```python
from build123d import *

# Parameters (mm, degrees)
SKETCH1_W                           = 3.81
SKETCH1_H                           = 63.5
CUT_EXTRUDE1_REACH                  = 281.224
CUT_EXTRUDE1_END_RADIUS             = 142.71625
SKETCH2_W                           = 1.524
SKETCH2_H                           = 38.1
CUT_EXTRUDE1_DIRECTION_2_REACH      = 281.224
CUT_EXTRUDE1_DIRECTION_2_END_RADIUS = 142.71625
CIRPATTERN1_COUNT                   = 4
CIRPATTERN1_ANGLE                   = 135


with BuildPart() as part:
    # Sketch1 → Revolve1 (revolve)
    with BuildSketch(Plane.XY, mode=Mode.PRIVATE) as revolve1_sk:
        with Locations((140.81125, 161.201652174)):
            Rectangle(SKETCH1_W, SKETCH1_H)
    revolve(revolve1_sk.sketch.rotate(Axis((0, 0, 0), (0, -1, 0)), 90), axis=Axis((0, 0, 0), (0, -1, 0)))

    # Cut-Extrude1: up to this cylinder (the profile starts inside it)
    cut_extrude1_end = Plane(origin=(0, 161.201652, 0), z_dir=(0, 1, 0)) * Cylinder(CUT_EXTRUDE1_END_RADIUS, 848.8805, mode=Mode.PRIVATE)
    # Sketch2 → Cut-Extrude1 (cut, up to the surface)
    with BuildSketch(Plane(origin=(0, 0, 0), x_dir=(0, 0, -1), z_dir=(1, 0, 0)), mode=Mode.PRIVATE) as cut_extrude1_sk1:
        with Locations((0, 161.201652174)):
            Rectangle(SKETCH2_W, SKETCH2_H)
    cut_extrude1_tool1 = extrude(cut_extrude1_sk1.sketch, amount=-CUT_EXTRUDE1_REACH, mode=Mode.PRIVATE) & cut_extrude1_end
    cut_extrude1 = cut_extrude1_tool1.solids().sort_by_distance((0, 161.201652, 0))[0]
    add(cut_extrude1, mode=Mode.SUBTRACT)

    # Cut-Extrude1 direction 2: up to this cylinder (the profile starts inside it)
    cut_extrude1_direction_2_end = Plane(origin=(0, 161.201652, 0), z_dir=(0, 1, 0)) * Cylinder(CUT_EXTRUDE1_DIRECTION_2_END_RADIUS, 848.8805, mode=Mode.PRIVATE)
    # Sketch2 → Cut-Extrude1 direction 2 (cut, up to the surface)
    with BuildSketch(Plane(origin=(0, 0, 0), x_dir=(0, 0, -1), z_dir=(1, 0, 0)), mode=Mode.PRIVATE) as cut_extrude1_direction_2_sk1:
        with Locations((0, 161.201652174)):
            Rectangle(SKETCH2_W, SKETCH2_H)
    cut_extrude1_direction_2_tool1 = extrude(cut_extrude1_direction_2_sk1.sketch, amount=CUT_EXTRUDE1_DIRECTION_2_REACH, mode=Mode.PRIVATE) & cut_extrude1_direction_2_end
    cut_extrude1_direction_2 = cut_extrude1_direction_2_tool1.solids().sort_by_distance((0, 161.201652, 0))[0]
    add(cut_extrude1_direction_2, mode=Mode.SUBTRACT)
    cut_extrude1 = cut_extrude1 + cut_extrude1_direction_2  # both directions under the feature's name, for the pattern or mirror that repeats it

    # CirPattern1: Cut-Extrude1 ×4 about axis
    cirpattern1_axis = Axis((0, 0, 0), (0, -1, 0))
    for i in range(1, CIRPATTERN1_COUNT):
        add(cut_extrude1.rotate(cirpattern1_axis, i * CIRPATTERN1_ANGLE / (CIRPATTERN1_COUNT - 1)), mode=Mode.SUBTRACT)


solid = part.part
```
Work out the finished part from the listing and answer in its coordinate system (mm). Give positions to 0.01 mm unless a question says otherwise; leave off trailing zeros. Loops run counter-clockwise (first coordinate to the right, second up) from the corner with the lowest first, then second, coordinate; pieces in that order, holes last. Notation, with made-up numbers: (-16, 14) - (9, 14) arc R23 cw to (9, 41) - close; hole circle Ø7 at (3.5, 21). An arc over 180 degrees is marked (long way). One line per question, with ' | ' between items.
(1) The part is cut by section A-A (y = 149). Count the separate pieces of the cut face and the enclosed holes in it, then the cut area to 3 significant figures.
Recorded:
separate pieces: 8 | enclosed holes: 0 | area: 3,320 mm²
(2) The part is cut by section C-C (x = -91). Write down the section's boundary in (y, z).
Recorded:
outline: (129.45, -109.94) - (192.95, -109.94) - (192.95, -104.95) - (129.45, -104.95) - close; (129.45, 104.95) - (192.95, 104.95) - (192.95, 109.94) - (129.45, 109.94) - close
(3) The mould has two halves that part along Z. Classify faces 1 (the face through (135.603, 161.646, -30.112)), 2 (the face through (54.661, 161.646, 131.834)), 3 (the face through (137, 129.452, -31)): +Z half, -Z half, draft (parallel to the pull), parting line (faces both ways), or undercut.
Recorded:
face 1: undercut | face 2: parting line | face 3: draft
(4) Each of these flat-tipped pins is pushed along its axis until it touches: pin 1 Ø3 at (x, y) = (-12, 146.5) entering from -Z; pin 2 Ø5 at (y, z) = (138.5, -67.5) entering from -X; pin 3 Ø12 at (y, z) = (162.5, -48) entering from -X. Where does it stop, or does it pass through?
Recorded:
pin 1: stops at z = -142.33 | pin 2: stops at x = -127.05 | pin 3: stops at x = -136.4
(5) Straight lines are drawn through the part: probe 1 along Z at (x, y) = (-28.5, 166.5); probe 2 along X at (y, z) = (142, -37.5); probe 3 along X at (y, z) = (158, -85). For each, find the intervals that lie inside material, in ascending order.
Recorded:
probe 1: z = -139.84 to -135.95, 135.95 to 139.84 | probe 2: x = -137.7 to -133.75, 133.75 to 137.7 | probe 3: x = -114.64 to -109.86, 109.86 to 114.64
(6) The part is cut by section B-B (z = -11). Write down the section's boundary in (x, y), then the cut area to 3 significant figures.
Recorded:
outline: (-142.29, 129.45) - (-138.47, 129.45) - (-138.47, 192.95) - (-142.29, 192.95) - close; (138.47, 129.45) - (142.29, 129.45) - (142.29, 192.95) - (138.47, 192.95) - close | area: 485 mm²
